from build123d import *

# Parameters (mm, degrees)
BOSS_EXTRUDE1_DEPTH = 10
FILLET1_R           = 1
FILLET2_R           = 0.5
FILLET3_R           = 1


with BuildPart() as part:
    # Sketch1 → Boss-Extrude1 (new body)
    with BuildSketch(Plane.XY):
        with BuildLine():
            Line((0.05, 14.37), (0.05, 4.504997225))
            ThreePointArc((0.05, 4.504997225), (0.993882062, 5.178181229), (2.05, 5.65641229))
            Line((2.05, 5.65641229), (2.05, 14.37))
            ThreePointArc((2.05, 14.37), (0.989726548, 16.929726548), (-1.57, 17.99))
            Line((-1.57, 17.99), (-2.748, 17.99))
            ThreePointArc((-2.748, 17.99), (-5.307726548, 16.929726548), (-6.368, 14.37))
            Line((-6.368, 14.37), (-4.368, 14.37))
            ThreePointArc((-4.368, 14.37), (-3.893512986, 15.515512986), (-2.748, 15.99))
            Line((-2.748, 15.99), (-1.57, 15.99))
            ThreePointArc((-1.57, 15.99), (-0.424487014, 15.515512986), (0.05, 14.37))
        make_face()
        with BuildLine():
            Line((0.05, -0.628490254), (0.05, -4.504997225))
            ThreePointArc((0.05, -4.504997225), (0.993882062, -5.178181229), (2.05, -5.65641229))
            Line((2.05, -5.65641229), (2.05, -3.477786652))
            ThreePointArc((2.05, -3.477786652), (0.721502268, -2.283720103), (0.05, -0.628490254))
        make_face()
        with BuildLine():
            ThreePointArc((2.05, 5.65641229), (0.993882062, 5.178181229), (0.05, 4.504997225))
            Line((0.05, 4.504997225), (0.05, 0.628490254))
            ThreePointArc((0.05, 0.628490254), (0.721502268, 2.283720103), (2.05, 3.477786652))
            Line((2.05, 3.477786652), (2.05, 5.65641229))
        make_face()
        with BuildLine():
            Line((2.05, -3.477786652), (2.05, -5.65641229))
            ThreePointArc((2.05, -5.65641229), (7.453415588, -4.858111773), (9.95, 0))
            ThreePointArc((9.95, 0), (7.453415588, 4.858111773), (2.05, 5.65641229))
            Line((2.05, 5.65641229), (2.05, 3.477786652))
            ThreePointArc((2.05, 3.477786652), (5.993508112, 3.424361254), (7.95, 0))
            ThreePointArc((7.95, 0), (5.993508112, -3.424361254), (2.05, -3.477786652))
        make_face()
        with BuildLine():
            Line((-1.57, -15.99), (-2.748, -15.99))
            ThreePointArc((-2.748, -15.99), (-3.893512986, -15.515512986), (-4.368, -14.37))
            Line((-4.368, -14.37), (-6.368, -14.37))
            ThreePointArc((-6.368, -14.37), (-5.307726548, -16.929726548), (-2.748, -17.99))
            Line((-2.748, -17.99), (-1.57, -17.99))
            ThreePointArc((-1.57, -17.99), (0.989726548, -16.929726548), (2.05, -14.37))
            Line((2.05, -14.37), (2.05, -5.65641229))
            ThreePointArc((2.05, -5.65641229), (0.993882062, -5.178181229), (0.05, -4.504997225))
            Line((0.05, -4.504997225), (0.05, -14.37))
            ThreePointArc((0.05, -14.37), (-0.424487014, -15.515512986), (-1.57, -15.99))
        make_face()
    extrude(amount=BOSS_EXTRUDE1_DEPTH)

    # Fillet1
    fillet1_edges = [part.edges().sort_by_distance(p)[0] for p in [
        (0.05, -0.628490254, 5),
        (0.05, 0.628490254, 5),
    ]]
    fillet(fillet1_edges, radius=FILLET1_R)

    # Fillet2
    fillet2_edges = [part.edges().sort_by_distance(p)[0] for p in [
        (2.05, 5.65641229, 5),
        (2.05, -5.65641229, 5),
    ]]
    fillet(fillet2_edges, radius=FILLET2_R)

    # Fillet3
    fillet3_edges = [part.edges().sort_by_distance(p)[0] for p in [
        (-6.368, 14.37, 5),
        (-4.368, 14.37, 5),
        (-6.368, -14.37, 5),
        (-4.368, -14.37, 5),
    ]]
    fillet(fillet3_edges, radius=FILLET3_R - 0.0001)  # a hair under: the kernel refuses the full size


solid = part.part
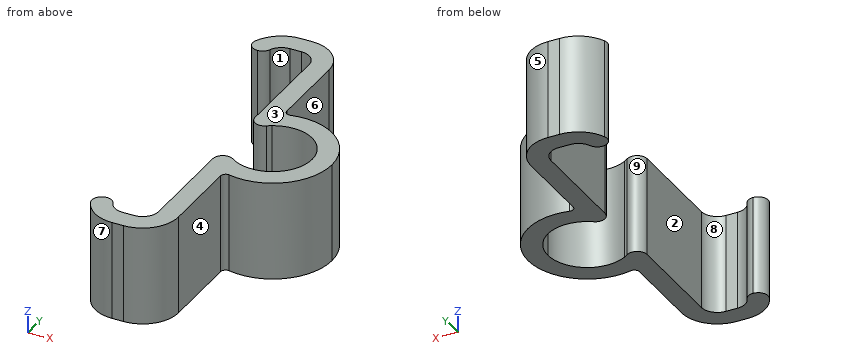
Could you check a few things on this model? Use its own coordinates, in mm. Face numbers are marked on the shaded views. A direction names the side the tool comes from. Give positions to 0.01 mm unless a question says otherwise; leave off trailing zeros. Order: outer loops, then holes, each group sorted by start corner. A loop starts at its lowest first (then second) coordinate and runs counter-clockwise, first axis right, second up. Notation, with made-up numbers: (-21.75, 86.5) - (-17.75, 86.5) arc R26 cw to (-17.75, 101.5) - close; hole circle Ø11 at (-20, 53.25). An arc over 180 degrees is marked (long way). Return JSON: item names as keys, results as strings. Group by question number.
Q1. Thinking about a two-plate mould opening in X: for the marked faces 6, 7, 8 and 9, which applies, pulls with the +X half, pulls with the -X half, needs draft (parallel to the pull), parting line crosses it, or undercut?
Q2. Please list where these lines run through material, in increasing order: line 1 along X through (y, z) = (-8.5, 9); line 2 along Y through (x, z) = (-4.5, 2.25); line 3 along X through (y, z) = (-15, 1.5). Write a range as [from, to].
Q3. Suppose I cut it at D-D, the plane y = 2.5. Please give me the cut outline in (x, z).
Q4. Suppose I cut it at C-C, the plane y = 7.5. Please give me the cut outline in (x, z), and give its area (3 significant figures).
Q5. Suppose I cut it at B-B, the plane x = 3.25. Please give me the cut outline in (y, z), and give its area (3 significant figures).
Q6. Which directions (+Z, -Z, +X, -X, +Y, -Y) give clear straight access to the entire face, cutting with the end or side of a thin tool? Please do the marked faces 1, 2, 3, 4 and 5.
Q7. Will these pins go through, and if not, where does the flat tip stop? pin 1 Ø1 at (x, y) = (1.5, -2.5) entering from +Z; pin 2 Ø3 at (x, z) = (-1, 1.5) entering from -Y; pin 3 Ø2 at (x, z) = (7, 6) entering from +Y; pin 4 Ø1 at (x, z) = (7.5, 1.5) entering from -Y.
Resolved:
{
 "1": {"face 6": "pulls with the +X half", "face 7": "pulls with the -X half", "face 8": "undercut", "face 9": "undercut"},
 "2": {"line 1": "x = [0.05, 2.05]", "line 2": "y = [-17.54, -14.63], [14.63, 17.54]", "line 3": "x = [-6.1, -4.24], [-0.08, 1.99]"},
 "3": {"outline": "(7.07, 0) - (9.4, 0) - (9.4, 10) - (7.07, 10) - close"},
 "4": {"outline": "(0.05, 0) - (2.05, 0) - (2.05, 10) - (0.05, 10) - close", "area": "20.0 mm2"},
 "5": {"outline": "(-5.93, 0) - (-3.91, 0) - (-3.91, 10) - (-5.93, 10) - close; (3.91, 0) - (5.93, 0) - (5.93, 10) - (3.91, 10) - close", "area": "40.5 mm2"},
 "6": {"face 1": "+Z, -Z", "face 2": "+Z, -Z, -X", "face 3": "+Z, +X, -X, +Y, -Y", "face 4": "+Z, -Z, +X, -Y", "face 5": "+Z, -Z, +X, +Y"},
 "7": {"pin 1": "passes through", "pin 2": "stops at y = -17.99", "pin 3": "stops at y = 5.62", "pin 4": "stops at y = -5.15"}
}
